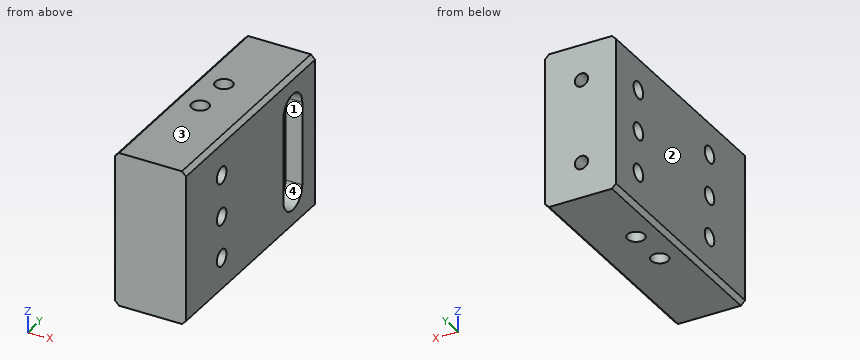
from build123d import *

# Parameters (mm, degrees)
SKETCH1_W           = 21.59
SKETCH1_H           = 46.99
BOSS_EXTRUDE1_DEPTH = 31.75
SKETCH2_R           = 2.6035
CUT_EXTRUDE1_DEPTH  = 47.99
SKETCH4_R           = 2.5527
CUT_EXTRUDE3_DEPTH  = 22.59
CUT_EXTRUDE5_DEPTH  = 5.08
SKETCH8_W           = 21.59
SKETCH8_H           = 46.99
BOSS_EXTRUDE2_DEPTH = 5.588
SKETCH9_R           = 2.0193
CUT_EXTRUDE6_DEPTH  = 5.08
SKETCH10_R          = 2.5527
CUT_EXTRUDE7_DEPTH  = 22.59
CHAMFER1_SIZE       = 1.27


with BuildPart() as part:
    # Sketch1 → Boss-Extrude1 (new body, symmetric)
    with BuildSketch(Plane(origin=(0, 0, 0), x_dir=(1, 0, 0), z_dir=(0, 1, 0))):
        Rectangle(SKETCH1_W, SKETCH1_H)
    extrude(amount=BOSS_EXTRUDE1_DEPTH, both=True)

    # Sketch2 → Cut-Extrude1 (cut, through all)
    with BuildSketch(Plane.XY.offset(23.495)):
        with Locations((-2.8956, 12.7)):
            Circle(SKETCH2_R)
        with Locations((-2.8956, 0)):
            Circle(SKETCH2_R)
    extrude(amount=-CUT_EXTRUDE1_DEPTH, mode=Mode.SUBTRACT)

    # Sketch4 → Cut-Extrude3 (cut, through all)
    with BuildSketch(Plane(origin=(10.795, 0, 0), x_dir=(0, 0, -1), z_dir=(1, 0, 0))):
        with Locations((-12.7, 25.4)):
            Circle(SKETCH4_R)
        with Locations((12.7, 25.4)):
            Circle(SKETCH4_R)
        with Locations((0, 25.4)):
            Circle(SKETCH4_R)
    extrude(amount=-CUT_EXTRUDE3_DEPTH, mode=Mode.SUBTRACT)

    # Sketch7 → Cut-Extrude5 (cut)
    with BuildSketch(Plane(origin=(10.795, 0, 0), x_dir=(0, 0, -1), z_dir=(1, 0, 0))):
        with BuildLine():
            Line((-12.7, 30.48), (12.7, 30.48))
            ThreePointArc((12.7, 30.48), (17.78, 25.4), (12.7, 20.32))
            Line((12.7, 20.32), (-12.7, 20.32))
            ThreePointArc((-12.7, 20.32), (-17.78, 25.4), (-12.7, 30.48))
        make_face()
    extrude(amount=-CUT_EXTRUDE5_DEPTH, mode=Mode.SUBTRACT)

    # Sketch8 → Boss-Extrude2 (add)
    with BuildSketch(Plane(origin=(0, 31.75, 0), x_dir=(1, 0, 0), z_dir=(0, 1, 0))):
        Rectangle(SKETCH8_W, SKETCH8_H)
    extrude(amount=BOSS_EXTRUDE2_DEPTH)

    # Sketch9 → Cut-Extrude6 (cut)
    with BuildSketch(Plane(origin=(0, 37.338, 0), x_dir=(1, 0, 0), z_dir=(0, 1, 0))):
        with Locations((-0.2794, 12.696926228)):
            Circle(SKETCH9_R)
        with Locations((-0.2794, -12.696926228)):
            Circle(SKETCH9_R)
    extrude(amount=-CUT_EXTRUDE6_DEPTH, mode=Mode.SUBTRACT)

    # Sketch10 → Cut-Extrude7 (cut, through all)
    with BuildSketch(Plane(origin=(10.795, 0, 0), x_dir=(0, 0, -1), z_dir=(1, 0, 0))):
        with Locations((0, -12.7)):
            Circle(SKETCH10_R)
        with Locations((12.7, -12.7)):
            Circle(SKETCH10_R)
        with Locations((-12.7, -12.7)):
            Circle(SKETCH10_R)
    extrude(amount=-CUT_EXTRUDE7_DEPTH, mode=Mode.SUBTRACT)

    # Chamfer1
    chamfer1_edges = [part.edges().sort_by_distance(p)[0] for p in [
        (10.795, 2.794, 23.495),
        (-10.795, 2.794, 23.495),
        (-10.795, 2.794, -23.495),
        (10.795, 2.794, -23.495),
    ]]
    chamfer(chamfer1_edges, length=CHAMFER1_SIZE)


solid = part.part
Geometry check sheet. Reference: the model listing, model coordinates, mm. Face numbers are marked on the shaded views. Round coordinates to 2 decimals unless told otherwise and drop trailing zeros. Order: outer loops, then holes, each group sorted by start corner. A loop starts at its lowest first (then second) coordinate and runs counter-clockwise, first axis right, second up. Notation, with made-up numbers: M 52,-22 L 66,-22 A30 cw 66,3 Z; hole C 77.5,48.25 d10. An arc over 180 degrees is marked long. Write each question's results on one line, items separated by ' | '. Start each with the question number.
1. Cross-section at A-A on z = 0. Give the number of separate pieces and of enclosed holes in the cut face, plus the area to 3 significant figures.
2. Material ranges on L1, parallel to Y at x = 8.5, z = 13; L2, parallel to Y at x = -5.25, z = 12; L3, parallel to Y at x = -4, z = 8, recorded low to high. Write a range as from..to.
3. Cross-section at C-C on y = 0. Record the boundary of the cut face in (x, z) (3 decimals), plus the area to 3 significant figures.
4. Cross-section at B-B on y = 25.4. Record the boundary of the cut face in (x, z) (3 decimals).
5. Go/stop test with flat-tipped pins: P1, Ø3.5, axis at x = -0.28, z = 12.7, coming from the +Y side; P2, Ø5, axis at y = 27.5, z = 5.5, coming from the +X side (3 decimals). Record where each tip stops, or that it passes through.
6. Draft check along Z on the marked faces 1, 2, 3 and 4. Enter one of: pulls with the +Z half, pulls with the -Z half, needs draft (parallel to the pull), parting line crosses it, or undercut.
Resolved:
1) separate pieces: 3 | enclosed holes: 2 | area: 1,200 mm2
2) L1: -31.75..-15.24, -10.16..20.33, 30.47..37.34 | L2: -31.75..-15.15, -10.25..-1.11, 1.11..11.59, 13.81..22.95, 27.85..37.34 | L3: -31.75..-2.36, 2.36..10.34, 15.06..37.34
3) outline: M -10.795,-22.225 L -9.525,-23.495 L -5.499,-23.495 L -5.499,23.495 L -9.525,23.495 L -10.795,22.225 Z; M -0.292,-23.495 L 9.525,-23.495 L 10.795,-22.225 L 10.795,22.225 L 9.525,23.495 L -0.292,23.495 Z | area: 767 mm2
4) outline: M -10.795,-22.225 L -9.525,-23.495 L 9.525,-23.495 L 10.795,-22.225 L 10.795,-17.78 L 5.715,-17.78 L 5.715,-15.253 L -10.795,-15.253 Z; M -10.795,-10.147 L 5.715,-10.147 L 5.715,-2.553 L -10.795,-2.553 Z; M -10.795,2.553 L 5.715,2.553 L 5.715,10.147 L -10.795,10.147 Z; M -10.795,15.253 L 5.715,15.253 L 5.715,17.78 L 10.795,17.78 L 10.795,22.225 L 9.525,23.495 L -9.525,23.495 L -10.795,22.225 Z
5) P1: y = 32.26 | P2: x = 5.715
6) face 1: undercut | face 2: needs draft | face 3: pulls with the +Z half | face 4: undercut
